The figure shows three views and two pictorial views of one solid part (mm, origin at its lowest corner). Answer the questions. Round coordinates to 2 decimals unless told otherwise and drop trailing zeros. Order: outer loops, then holes, each group sorted by start corner. A loop starts at its lowest first (then second) coordinate and runs counter-clockwise, first axis right, second up. Notation, with made-up numbers: (82.25, -12.75) -> (103.25, -12.75) arc R26 cw to (103.25, 6.25) -> close; hole circle Ø10 at (32, -6). An arc over 180 degrees is marked (long way). Answer as a JSON object with one key per item and string values. Group by question number.
Item 1: Section D-D, the plane y = 11 is taken. Write down the section's boundary in (x, z) (1 decimal), plus the area to 3 significant figures.
Item 2: Consider probe 1 along Z at (x, y) = (25, 42.25) (1 decimal); probe 2 along X at (y, z) = (16.5, 17.75) (1 decimal); probe 3 along Y at (x, z) = (22.5, 12.5) (1 decimal). Determine where each line is inside the solid, lowest interval first. Write a range as from..to.
Item 3: Section A-A, the plane x = 25 is taken. Write down the section's boundary in (y, z) (1 decimal).
Item 4: Section C-C, the plane z = 9.25 is taken. Count the separate pieces of the cut face and the enclosed holes in it, plus the area to 3 significant figures.
Item 5: Given P1, Ø1.5, axis at x = 28, y = 35, coming from the -Z side; P2, Ø6, axis at x = 8.5, z = 12, coming from the -Y side; P3, Ø8, axis at y = 18.5, z = 17, coming from the -X side (1 decimal); P4, Ø5, axis at y = 45, z = 13, coming from the -X side (1 decimal), each flat-ended and moving along its own axis, determine where each tip first touches the part or whether it passes through.
Item 6: Section B-B, the plane z = 5 is taken. Write down the section's boundary in (x, y) (1 decimal).
Item 7: The mould has two halves that part along Z. Classify the marked faces 1, 2 and 3: pulls with the +Z half, pulls with the -Z half, needs draft (parallel to the pull), parting line crosses it, or undercut.
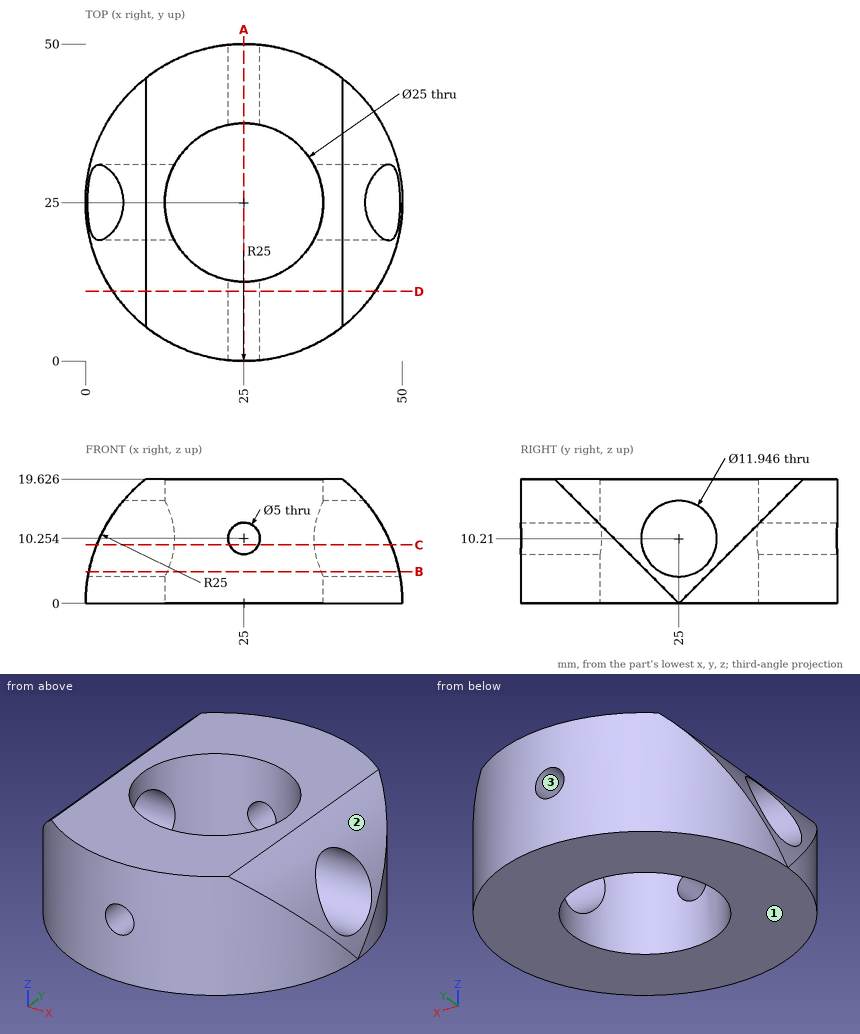
Values found:
{
 "1": {"outline": "(4.3, 0) -> (45.7, 0) -> (45.7, 14) arc R25 ccw to (40.5, 19.6) -> (9.5, 19.6) arc R25 ccw to (4.3, 14) -> close; hole circle Ø5 at (25, 10.3)", "area": "767 mm2"},
 "2": {"probe 1": "0..7.8, 12.8..19.6", "probe 2": "7.4..15.8, 34.2..42.6", "probe 3": "0.1..12.8, 37.2..49.9"},
 "3": {"outline": "(0, 0) -> (12.5, 0) -> (12.5, 7.8) -> (0, 7.8) -> close; (0, 12.8) -> (12.5, 12.8) -> (12.5, 19.6) -> (0, 19.6) -> close; (37.5, 0) -> (50, 0) -> (50, 7.8) -> (37.5, 7.8) -> close; (37.5, 12.8) -> (50, 12.8) -> (50, 19.6) -> (37.5, 19.6) -> close"},
 "4": {"separate pieces": "4", "enclosed holes": "0", "area": "1,050 mm2"},
 "5": {"P1": "through", "P2": "y = 3.96", "P3": "x = 3.6", "P4": "x = 7.1"},
 "6": {"outline": "(0.5, 20) arc R25 ccw to (49.5, 20) -> (49.5, 22.1) -> (37.2, 22.1) arc R12.5 cw to (12.8, 22.1) -> (0.5, 22.1) -> close; (0.5, 27.9) -> (12.8, 27.9) arc R12.5 cw to (37.2, 27.9) -> (49.5, 27.9) -> (49.5, 30) arc R25 ccw to (0.5, 30) -> close"},
 "7": {"face 1": "pulls with the -Z half", "face 2": "pulls with the +Z half", "face 3": "undercut"}
}
